Design review of the part built by this model. Coordinates are the model's own, in mm. Give positions to 0.01 mm unless a question says otherwise; leave off trailing zeros. Loops run counter-clockwise (first coordinate to the right, second up) from the corner with the lowest first, then second, coordinate; pieces in that order, holes last. Notation, with made-up numbers: (61, 43) -> (110, 43) arc R28 cw to (110, 73) -> close; hole circle Ø3 at (-11, -20.75). An arc over 180 degrees is marked (long way). Use CSV: the item, a comma, the result in double quotes. Start each with the question number.
Item 1: Clearance check with flat-ended pins moving along their axes: pin 1 (4.5 mm diameter, centred on x = 0, z = 0, fed in from +Y); pin 2 (1.5 mm diameter, centred on y = 1, z = 6, fed in from -X). State where each tip first meets the part, or that it passes through.
Item 2: Wall thickness on line 1 along Z through (x, y) = (-0.25, 2); line 2 along X through (y, z) = (-0.35, 0.5); line 3 along X through (y, z) = (-0.85, -5): over which ranges is each line inside the solid? List them lowest first. Write a range as from..to.
Item 3: We need section D-D (y = -0.6). State the section outline as (x, z) points, plus the area to 3 significant figures.
Item 4: The part is to be moulded in two halves that separate along Y. For faces 1 (the face through (-1.65, -0.12, -7.44)), 2 (the face through (2, -2.5, -2)), 3 (the face through (2, 2.5, -2)), say which applies: +Y half, -Y half, draft (parallel to the pull), parting line (faces both ways), or undercut.
Item 5: We need section C-C (y = 1.65). State the section outline as (x, z) points, plus the area to 3 significant figures.
from build123d import *

# Parameters (mm, degrees)
F0_R     = 10
F0_R_2   = 2.5
F1_DEPTH = 2.5
F2_SIZE  = 2.49999


# Not quite as in the source:
# - a fillet or chamfer is up to 0.001 mm smaller than in the source, because OpenCascade refuses the exact size


with BuildPart() as f1:
    # F0 (on Front) → F1 (new body)
    with BuildSketch(Plane.XZ):
        Circle(F0_R)
        Circle(F0_R_2, mode=Mode.SUBTRACT)
    extrude(amount=F1_DEPTH)

    # F2 (size 2.5 in the source; OpenCascade refuses exactly that, so slightly less here)
    f2_edges = [f1.edges().sort_by_distance(p)[0] for p in [
        (-10, 0, 0),
    ]]
    chamfer(f2_edges, length=F2_SIZE)

    # F3: F1 across plane


with BuildPart() as f1_1:
    add(f1.part)
    add(f1.part.mirror(Plane.XZ))


solid = f1_1.part
Results found:
1,pin 1,"through"
1,pin 2,"x = -7.22"
2,line 1,"-9.5..-2.49, 2.49..9.5"
2,line 2,"-7.83..-2.45, 2.45..7.83"
2,line 3,"-6.69..6.69"
3,outline,"circle Ø16.2 at (0, 0); hole circle Ø5 at (0, 0)"
3,area,"186 mm²"
4,face 1,"undercut"
4,face 2,"-Y half"
4,face 3,"+Y half"
5,outline,"circle Ø18.3 at (0, 0); hole circle Ø5 at (0, 0)"
5,area,"243 mm²"
